from build123d import *

# Parameters (mm, degrees)
BOSS_EXTRU_1_DEPTH = 31.5
ESQUISSE2_R        = 15
BOSS_EXTRU_2_DEPTH = 50


with BuildPart() as part:
    # Esquisse1 → Boss.-Extru.1 (new body)
    with BuildSketch(Plane.XY):
        with BuildLine():
            Line((35, 26), (76, 26))
            Line((76, 26), (76, 0))
            Line((76, 0), (0, 0))
            Line((0, 0), (0, 26))
            Line((0, 26), (5, 26))
            ThreePointArc((5, 26), (20, 41), (35, 26))
        make_face()
    extrude(amount=BOSS_EXTRU_1_DEPTH)

    # Esquisse2 → Boss.-Extru.2 (add)
    with BuildSketch(Plane(origin=(0, 26, 0), x_dir=(1, 0, 0), z_dir=(0, 1, 0))):
        with Locations((54, -15.75)):
            Circle(ESQUISSE2_R)
    extrude(amount=BOSS_EXTRU_2_DEPTH)


solid = part.part
Check sheet for the modelled part. Datum: model origin and axes. Units: mm. A direction names the side the tool comes from. Coordinates: 2 decimals unless noted, no trailing zeros. Loops run counter-clockwise (first coordinate to the right, second up) from the corner with the lowest first, then second, coordinate; pieces in that order, holes last. Notation, with made-up numbers: (68.25, -2) -> (101.25, -2) arc R20 cw to (101.25, 13) -> close; hole circle Ø6 at (17, 69). An arc over 180 degrees is marked (long way). Answer in a Markdown table with one row per item.
1. Sectioned sample at B-B, the plane z = 15.75. Record the boundary of the cut face in (x, y).
Check values:
| item | result |
|---|---|
| outline | (0, 0) -> (76, 0) -> (76, 26) -> (69, 26) -> (69, 76) -> (39, 76) -> (39, 26) -> (35, 26) arc R15 ccw to (5, 26) -> (0, 26) -> close |
2. Material ranges on line 1 along Z through (x, y) = (54.5, 58.5); line 2 along X through (y, z) = (29, 16.5); line 3 along X through (y, z) = (34.5, 14.5), recorded low to high. Write a range as [from, to].
Check values:
| item | result |
|---|---|
| line 1 | z = [0.76, 30.74] |
| line 2 | x = [5.3, 34.7], [39.02, 68.98] |
| line 3 | x = [7.64, 32.36], [39.05, 68.95] |
3. Sectioned sample at A-A, the plane y = 35. Record the boundary of the cut face in (x, z).
Check values:
| item | result |
|---|---|
| outline | (8, 0) -> (32, 0) -> (32, 31.5) -> (8, 31.5) -> close; circle Ø30 at (54, 15.75) |
4. Sectioned sample at C-C, the plane x = 54. Record the boundary of the cut face in (y, z), then the cut area to 3 significant figures.
Check values:
| item | result |
|---|---|
| outline | (0, 0) -> (26, 0) -> (26, 0.75) -> (76, 0.75) -> (76, 30.75) -> (26, 30.75) -> (26, 31.5) -> (0, 31.5) -> close |
| area | 2,320 mm2 |
5. Release check for a two-part mould opening along X. For faces 3 (the face through (2, 26, 16)), 4 (the face through (0, 13, 16)), 5 (the face through (69, 26, 12)), 6 (the face through (76, 13, 16)) record: released by +X, released by -X, zero draft, split by the parting line, or undercut.
Check values:
| item | result |
|---|---|
| face 3 | zero draft |
| face 4 | released by -X |
| face 5 | undercut |
| face 6 | released by +X |
6. Access from +Z, -Z, +X, -X, +Y, -Y to the whole of each face (thin tool, end or side, straight path). Record for faces 1 (the face through (39, 16, 0)), 2 (the face through (42.944, 50.65, 5.612)).
Check values:
| item | result |
|---|---|
| face 1 | -Z, +X, -X, +Y, -Y |
| face 2 | +Y |
7. Sectioned sample at D-D, the plane y = 55. Record the boundary of the cut face in (x, z), then the cut area to 3 significant figures.
Check values:
| item | result |
|---|---|
| outline | circle Ø30 at (54, 15.75) |
| area | 707 mm2 |
8. Go/stop test with flat-tipped pins: pin 1 (8 mm diameter, centred on y = 51.5, z = 9.5, fed in from -X); pin 2 (4 mm diameter, centred on y = 66.5, z = 19, fed in from -X); pin 3 (6 mm diameter, centred on y = 54, z = 25.5, fed in from -X). Record where each tip stops, or that it passes through.
Check values:
| item | result |
|---|---|
| pin 1 | stops at x = 39.17 |
| pin 2 | stops at x = 39.05 |
| pin 3 | stops at x = 40.6 |
